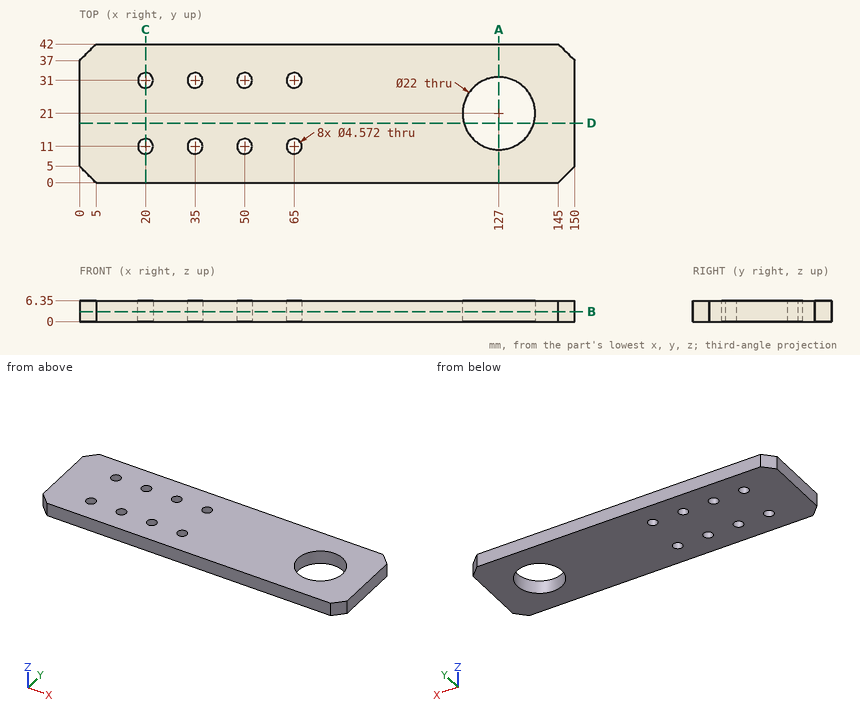
The figure shows three views and two pictorial views of one solid part (mm, origin at its lowest corner). Answer the questions. Give positions to 0.01 mm unless a question says otherwise; leave off trailing zeros. Loops run counter-clockwise (first coordinate to the right, second up) from the corner with the lowest first, then second, coordinate; pieces in that order, holes last. Notation, with made-up numbers: (31, 6.5) -> (67, 6.5) arc R18 ccw to (67, 19.5) -> close; hole circle Ø4 at (-10.5, 43.25). An arc over 180 degrees is marked (long way). Use a Markdown table: item, result. Add a question column.
1. Find the intervals of material crossed by probe 1 along Y at (x, z) = (35, 2.5); probe 2 along Y at (x, z) = (36, 4); probe 3 along Y at (x, z) = (127, 4), in increasing order.
2. Section D-D on y = 18 is taken. Determine the outline of the cut face in (x, z), and give its area (3 significant figures).
3. Section C-C on x = 20 is taken. Determine the outline of the cut face in (y, z).
4. Section A-A on x = 127 is taken. Determine the outline of the cut face in (y, z).
5. Section B-B on z = 3 is taken. State how many separate pieces and enclosed holes the cut face has, and give its area (3 significant figures).
6. A flat-ended cylindrical pin translates along its axis: pin 1 Ø2.5 at (x, y) = (50, 31) entering from +Z. Find the tip coordinate at first contact, or state that the pin passes through.
Results below:
| question | item | result |
|---|---|---|
| 1 | probe 1 | y = 0 to 8.71, 13.29 to 28.71, 33.29 to 42 |
| 1 | probe 2 | y = 0 to 8.94, 13.06 to 28.94, 33.06 to 42 |
| 1 | probe 3 | y = 0 to 10, 32 to 42 |
| 2 | outline | (0, 0) -> (116.42, 0) -> (116.42, 6.35) -> (0, 6.35) -> close; (137.58, 0) -> (150, 0) -> (150, 6.35) -> (137.58, 6.35) -> close |
| 2 | area | 818 mm^2 |
| 3 | outline | (0, 0) -> (8.71, 0) -> (8.71, 6.35) -> (0, 6.35) -> close; (13.29, 0) -> (28.71, 0) -> (28.71, 6.35) -> (13.29, 6.35) -> close; (33.29, 0) -> (42, 0) -> (42, 6.35) -> (33.29, 6.35) -> close |
| 4 | outline | (0, 0) -> (10, 0) -> (10, 6.35) -> (0, 6.35) -> close; (32, 0) -> (42, 0) -> (42, 6.35) -> (32, 6.35) -> close |
| 5 | separate pieces | 1 |
| 5 | enclosed holes | 9 |
| 5 | area | 5,740 mm^2 |
| 6 | pin 1 | passes through |
